from build123d import *

# Parameters (mm, degrees)
SKETCH1_W           = 80
SKETCH1_H           = 50
BOSS_EXTRUDE1_DEPTH = 20
CUT_EXTRUDE1_REACH  = 22
SKETCH2_R           = 20.5


with BuildPart() as part:
    # Sketch1 → Boss-Extrude1 (new body)
    with BuildSketch(Plane(origin=(0, 2495.407712162, 0), x_dir=(1, 0, 0), z_dir=(0, 1, 0))):
        with Locations((-32.832129773, 17.792108153)):
            Rectangle(SKETCH1_W, SKETCH1_H)
    extrude(amount=BOSS_EXTRUDE1_DEPTH)

    # Sketch2 → Cut-Extrude1 (cut, up to next)
    with BuildSketch(Plane.XZ.offset(-2495.407712162), mode=Mode.PRIVATE) as cut_extrude1_sk1:
        with Locations((-32.832129773, -17.792108153)):
            Circle(SKETCH2_R)
    cut_extrude1_tool1 = extrude(cut_extrude1_sk1.sketch, amount=-CUT_EXTRUDE1_REACH, mode=Mode.PRIVATE) & part.part
    add(cut_extrude1_tool1.solids().sort_by_distance((-32.83213, 2495.407712, -17.792108))[0], mode=Mode.SUBTRACT)


solid = part.part
For this review, take the finished solid that the model builds, in its own axes (mm). Coordinates: 2 decimals unless noted, no trailing zeros. Loops run counter-clockwise (first coordinate to the right, second up) from the corner with the lowest first, then second, coordinate; pieces in that order, holes last. Notation, with made-up numbers: (77, 76.5) - (110, 76.5) arc R21 cw to (110, 110.5) - close; hole circle Ø7 at (63.25, 66). An arc over 180 degrees is marked (long way). Use a Markdown table: item, result. Add a question column.
Item 1: We need section A-A (z = -11.5). Give the boundary of the cut face in (x, y), and give its area (3 significant figures).
Item 2: For line 1 (Z direction, x = -40, y = 2511.5); line 2 (X direction, y = 2501.75, z = -3.5); line 3 (X direction, y = 2511.5, z = -3), list the stretches that pass through material, from the lowest coordinate up.
Item 3: We need section B-B (x = -18). Give the boundary of the cut face in (y, z), and give its area (3 significant figures).
Item 4: Mouldability with a two-part tool opening along X and no side actions: class faces 1 (the face through (-49.1, 2505.268, -30.266)), 2 (the face through (-33, 2505, 7.208)), 3 (the face through (-72.832, 2505, -17)) as pulls with the +X half, pulls with the -X half, needs draft (parallel to the pull), parting line crosses it, or undercut.
Item 5: We need section C-C (y = 2501.5). Give the boundary of the cut face in (x, z).
Results list:
| question | item | result |
|---|---|---|
| 1 | outline | (-72.83, 2495.41) - (-52.34, 2495.41) - (-52.34, 2515.41) - (-72.83, 2515.41) - close; (-13.32, 2495.41) - (7.17, 2495.41) - (7.17, 2515.41) - (-13.32, 2515.41) - close |
| 1 | area | 820 mm^2 |
| 2 | line 1 | z = -42.79 to -37, 1.41 to 7.21 |
| 2 | line 2 | x = -72.83 to -47.53, -18.14 to 7.17 |
| 2 | line 3 | x = -72.83 to -47.03, -18.64 to 7.17 |
| 3 | outline | (2495.41, -42.79) - (2515.41, -42.79) - (2515.41, -31.94) - (2495.41, -31.94) - close; (2495.41, -3.64) - (2515.41, -3.64) - (2515.41, 7.21) - (2495.41, 7.21) - close |
| 3 | area | 434 mm^2 |
| 4 | face 1 | undercut |
| 4 | face 2 | needs draft |
| 4 | face 3 | pulls with the -X half |
| 5 | outline | (-72.83, -42.79) - (7.17, -42.79) - (7.17, 7.21) - (-72.83, 7.21) - close; hole circle Ø41 at (-32.83, -17.79) |
